```python
from build123d import *

# Parameters (mm, degrees)
BOSS_EXTRU_1_DEPTH = 1.4
CONG_1_R           = 1


with BuildPart() as part:
    # Esquisse1 → Boss.-Extru.1 (new body)
    with BuildSketch(Plane(origin=(0, 0, 0), x_dir=(0, 1, 0), z_dir=(0, 0, 1))):
        with BuildLine():
            ThreePointArc((1.8, 0), (-0.9, -1.558845727), (-0.9, 1.558845727))
            Line((-0.9, 1.558845727), (-2.5, 4.330127019))
            ThreePointArc((-2.5, 4.330127019), (-2.5, -4.330127019), (5, 0))
            ThreePointArc((5, 0), (4.330127019, 2.5), (2.5, 4.330127019))
            Line((2.5, 4.330127019), (0.9, 1.558845727))
            ThreePointArc((0.9, 1.558845727), (1.558845727, 0.9), (1.8, 0))
        make_face()
    extrude(amount=BOSS_EXTRU_1_DEPTH)

    # Congé1
    cong_1_edges = [part.edges().sort_by_distance(p)[0] for p in [
        (-1.558845727, -0.9, 0.7),
        (-1.558845727, 0.9, 0.7),
        (-4.330127019, 2.5, 0.7),
        (-4.330127019, -2.5, 0.7),
    ]]
    fillet(cong_1_edges, radius=CONG_1_R)


solid = part.part
```
Model file for the job. Use its own axes, mm. A direction names the side the tool comes from. Coordinates: 2 decimals unless noted, no trailing zeros. Loops run counter-clockwise (first coordinate to the right, second up) from the corner with the lowest first, then second, coordinate; pieces in that order, holes last. Notation, with made-up numbers: (-23.75, 6) -> (-10.75, 6) arc R34 ccw to (-10.75, 39) -> close; hole circle Ø4 at (16.5, -18). An arc over 180 degrees is marked (long way). Answer as a JSON object with one key per item and string values.
Q1. Cut at A-A (x = -0.5). List the corners of the cut face in (y, z), and give its area (3 significant figures).
Report:
{"outline": "(-4.97, 0) -> (-1.73, 0) -> (-1.73, 1.4) -> (-4.97, 1.4) -> close; (1.73, 0) -> (4.97, 0) -> (4.97, 1.4) -> (1.73, 1.4) -> close", "area": "9.09 mm2"}
Q2. Flat gauge pin, fed straight in: P1, Ø5, axis at x = -1.5, y = -1.5, coming from the -Z side. Where does the tip first touch, or does it go through?
Report:
{"P1": "stops at z = 0"}
Q3. 3-axis set-ups, long thin cutter, end or side, ignore diameter. For faces 1 (the flat face through (-2.802, -1.618, 0.69)), 2 (the cylindrical face through (-1.677, -1.178, 0.71)), 3 (the flat face through (2, 0, 1.4)): which of +Z, -Z, +X, -X, +Y, -Y reach the whole face in a straight line?
Report:
{"face 1": "+Z, -Z, -X", "face 2": "+Z, -Z", "face 3": "+Z, +X, -X, +Y, -Y"}
Q4. Probe probe 1 along Y at (x, z) = (0, 0.6); probe 2 along X at (y, z) = (0, 1.05); probe 3 along Y at (x, z) = (-2, 0.7). List the from-to ranges inside material, lowest first.
Report:
{"probe 1": "y = -5 to -1.8, 1.8 to 5", "probe 2": "x = 1.8 to 5", "probe 3": "y = -4.58 to -1.2, 1.2 to 4.58"}
Q5. Pull direction Y, two halves, no side cores. Call faces 4 (the cylindrical face through (-3.847, 2.68, 0.71)), 5 (the flat face through (2, 0, 0)), 6 (the cylindrical face through (-1.694, 1.176, 0.71)): released by +Y, released by -Y, zero draft, split by the parting line, or undercut.
Report:
{"face 4": "undercut", "face 5": "zero draft", "face 6": "undercut"}
Q6. Cut at B-B (z = 1.2). List the corners of the cut face in (x, y), and give its area (3 significant figures).
Report:
{"outline": "(-3.57, -3.5) arc R5 ccw (long way) to (-3.57, 3.5) arc R1 ccw to (-3.35, 1.94) -> (-2.26, 1.31) arc R1 ccw to (-1.13, 1.4) arc R1.8 cw (long way) to (-1.13, -1.4) arc R1 ccw to (-2.26, -1.31) -> (-3.35, -1.94) arc R1 ccw to start", "area": "56.1 mm2"}
Q7. Cut at D-D (x = -2.5). List the corners of the cut face in (y, z).
Report:
{"outline": "(-4.33, 0) -> (-1.44, 0) -> (-1.44, 1.4) -> (-4.33, 1.4) -> close; (1.44, 0) -> (4.33, 0) -> (4.33, 1.4) -> (1.44, 1.4) -> close"}
Q8. Cut at C-C (y = 0). List the corners of the cut face in (x, z), and give its area (3 significant figures).
Report:
{"outline": "(1.8, 0) -> (5, 0) -> (5, 1.4) -> (1.8, 1.4) -> close", "area": "4.48 mm2"}
